Autodesk Inventor part; units mm, degrees
ref_plane "YZ Plane" through (0, 0, 0) normal (1, 0, 0) x (0, 1, 0)
ref_plane "XZ Plane" through (0, 0, 0) normal (0, 1, 0) x (-1, 0, 0)
ref_plane "XY Plane" through (0, 0, 0) normal (0, 0, 1) x (1, 0, 0)
sketch "Esboço1" plane through (0, 0, 0) normal (0, 0, 1) x (1, 0, 0)
  line L0 (0, 0) -> (9, 0)
  line L1 (9, 0) -> (9, 6.65)
  line L2 (9, 6.65) -> (0, 6.65)
  line L3 (0, 6.65) -> (0, 4.65)
  line L4 (0, 4.65) -> (2.5, 4.65)
  line L5 (2.5, 4.65) -> (2.5, 0)
  dimension "d0" = 9
  dimension "d1" = 6.65
  dimension "d2" = 2
  dimension "d3" = 2.5
revolve "Revolução1" add sketch "Esboço1" angle 360 about axis through (0, 0, 0) along (1, 0, 0)
sketch "Esboço2" plane through (9, 0, 0) normal (1, 0, 0) x (0, 0, -1)
  circle A0 centre (0, 0) radius 2
  dimension "d5" = 4
extrude "Extrusão1" add sketch "Esboço2" along normal blind 1.5
sketch "Esboço3" plane through (2.5, 0, 0) normal (-1, 0, 0) x (0, 0, 1)
  circle A0 centre (0, 0) radius 1.5
  dimension "d8" = 3
extrude "Extrusão2" cut sketch "Esboço3" against normal blind 4
sketch "Esboço4" plane through (0, 0, 0) normal (-1, 0, 0) x (0, 0, 1)
  point P0 (0, 0)
sketch "Esboço5" plane through (9, 0, 0) normal (1, 0, 0) x (0, 0, -1)
  point P0 (0, 0)
sketch "Esboço6" plane through (10.5, 0, 0) normal (1, 0, 0) x (0, 0, -1)
  circle A0 centre (0, 0) radius 2
  circle A1 centre (0, 0) radius 1
  dimension "d11" = 2
extrude "Extrusão3" cut sketch "Esboço6" against normal blind 1.06 contours A1
Geometry: final body of the model. Coordinates: model frame, mm. A direction names the side the tool comes from. Round coordinates to 2 decimals unless told otherwise and drop trailing zeros. Write each loop counter-clockwise with the first axis right and the second up, starting at its lowest first coordinate (ties: lowest second). Pieces come first, ordered by that corner, then holes.
Item 1: Pin query (flat end, axial travel): P1, Ø1.5, axis at y = 0, z = 0.5, coming from the -X side; P2, Ø3, axis at x = 3.5, z = 3, coming from the -Y side; P3, Ø4.5, axis at y = -1, z = 2, coming from the -X side; P4, Ø1.6, axis at y = 0, z = -0.5, coming from the +X side. Return the tip coordinate at first contact, or that it passes through.
Item 2: Material intervals for L1, parallel to Z at x = 1.5, y = 0; L2, parallel to Y at x = 10, z = 0; L3, parallel to X at y = -5.25, z = -3.75, sorted ascending.
Item 3: Set-up query: faces 4 (the face through (1.27, 2.5, 3.92)), 5 (the face through (10, -1, 0)), 6 (the face through (0, -5, -1)). Return all of +Z, -Z, +X, -X, +Y, -Y with unobstructed straight access to the full face (end or side cutting, diameter ignored); none if empty.
Item 4: Mould query, pull axis Y, two halves, no side actions, for faces 1 (the face through (4.44, 3.07, 5.9)), 2 (the face through (9.44, 0, 0)), 3 (the face through (10.5, -1, -1)). Classes: +Y half, -Y half, draft (parallel to the pull), parting line (faces both ways), or undercut.
Item 5: Section query A-A (z = 0). Return loops of the section in (x, y).
Item 6: Section query D-D (z = 3.5). Return loops of the section in (x, y), plus the area to 3 significant figures.
Item 7: Section query C-C (x = 6). Return loops of the section in (y, z), plus the area to 3 significant figures.
Completed:
1. P1: stops at x = 6.5
1. P2: stops at y = -6.48
1. P3: stops at x = 2.5
1. P4: stops at x = 10.5
2. L1: z = -6.65 to -4.65, 4.65 to 6.65
2. L2: y = -2 to -1, 1 to 2
2. L3: x = 0 to 9
3. face 4: -X
3. face 5: +X
3. face 6: +Z, -Z, -X, +Y, -Y
4. face 1: parting line
4. face 2: undercut
4. face 3: draft
5. outline: (0, -6.65) - (9, -6.65) - (9, -2) - (10.5, -2) - (10.5, -1) - (9.44, -1) - (9.44, 1) - (10.5, 1) - (10.5, 2) - (9, 2) - (9, 6.65) - (0, 6.65) - (0, 4.65) - (2.5, 4.65) - (2.5, 1.5) - (6.5, 1.5) - (6.5, -1.5) - (2.5, -1.5) - (2.5, -4.65) - (0, -4.65) - close
6. outline: (0, -5.65) - (9, -5.65) - (9, 5.65) - (0, 5.65) - (0, 3.06) - (2.5, 3.06) - (2.5, -3.06) - (0, -3.06) - close
6. area: 86.5 mm2
7. outline: circle Ø13.3 at (0, 0); hole circle Ø3 at (0, 0)
7. area: 132 mm2
